Design review of the part shown in the three views and the two pictorial views. Dimensions are in mm from the part's minimum x, y and z. A direction names the side the tool comes from. Round coordinates to 2 decimals unless told otherwise and drop trailing zeros. Write each loop counter-clockwise with the first axis right and the second up, starting at its lowest first coordinate (ties: lowest second). Pieces come first, ordered by that corner, then holes. Notation, with made-up numbers: (6.5, 72.25) -> (32.5, 72.25) arc R34 cw to (32.5, 104.25) -> close; hole circle Ø1 at (40, 84). An arc over 180 degrees is marked (long way). One line per question, with ' | ' between items. Start each with the question number.
1) Insertion check: pin 1 Ø1 at (x, z) = (16.5, 6) entering from -Y; pin 2 Ø3 at (x, z) = (12.5, 1.5) entering from -Y; pin 3 Ø4 at (y, z) = (2, 4.5) entering from +X. Each pin has a flat end and moves straight along its axis. Give the tip position at first contact, or say it passes through.
2) Consider section A-A (x = 10.43). Give the boundary of the cut face in (y, z), then the cut area to 3 significant figures.
3) Consider section B-B (y = 6.25). Give the boundary of the cut face in (x, z), then the cut area to 3 significant figures.
4) Consider section D-D (x = 2.81). Give the boundary of the cut face in (y, z).
5) Consider section C-C (z = 2.5). Give the boundary of the cut face in (x, y).
6) For the marked faces 1 and 2, list the 3-axis set-ups (+Z, -Z, +X, -X, +Y, -Y) from which the entire face can be reached by the end or side of a thin tool; tool diameter is ignored.
7) For probe 1 along Y at (x, z) = (7.5, 3); probe 2 along X at (y, z) = (5.75, 11); probe 3 along Z at (x, y) = (24, 11.25), list the stretches that pass through material, from the lowest coordinate up.
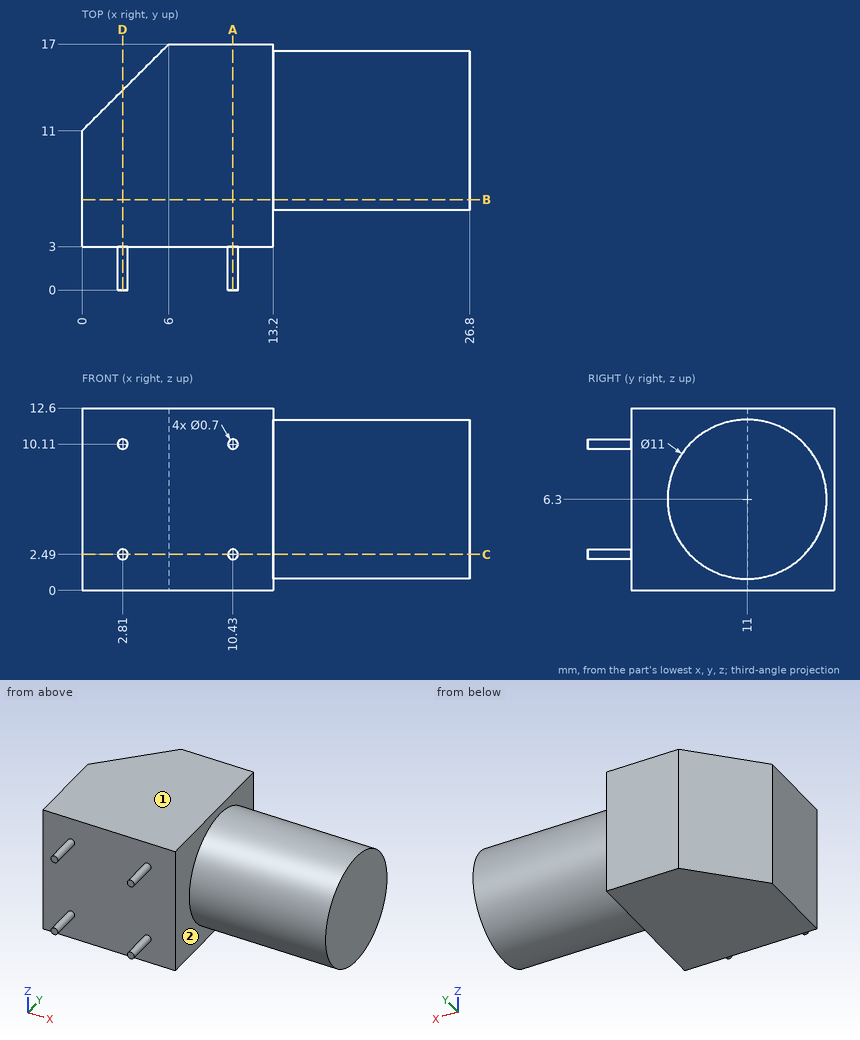
From the geometry:
1) pin 1: stops at y = 5.5 | pin 2: stops at y = 3 | pin 3: stops at x = 13.2
2) outline: (0, 2.14) -> (3, 2.14) -> (3, 0) -> (17, 0) -> (17, 12.6) -> (3, 12.6) -> (3, 10.46) -> (0, 10.46) -> (0, 9.76) -> (3, 9.76) -> (3, 2.84) -> (0, 2.84) -> close | area: 181 mm2
3) outline: (0, 0) -> (13.2, 0) -> (13.2, 3.53) -> (26.8, 3.53) -> (26.8, 9.07) -> (13.2, 9.07) -> (13.2, 12.6) -> (0, 12.6) -> close | area: 242 mm2
4) outline: (0, 2.14) -> (3, 2.14) -> (3, 0) -> (13.81, 0) -> (13.81, 12.6) -> (3, 12.6) -> (3, 10.46) -> (0, 10.46) -> (0, 9.76) -> (3, 9.76) -> (3, 2.84) -> (0, 2.84) -> close
5) outline: (0, 3) -> (2.46, 3) -> (2.46, 0) -> (3.16, 0) -> (3.16, 3) -> (10.08, 3) -> (10.08, 0) -> (10.78, 0) -> (10.78, 3) -> (13.2, 3) -> (13.2, 7.02) -> (26.8, 7.02) -> (26.8, 14.98) -> (13.2, 14.98) -> (13.2, 17) -> (6, 17) -> (0, 11) -> close
6) face 1: +Z, +X, -X, +Y, -Y | face 2: +X
7) probe 1: y = 3 to 17 | probe 2: x = 0 to 13.2 | probe 3: z = 0.81 to 11.79
